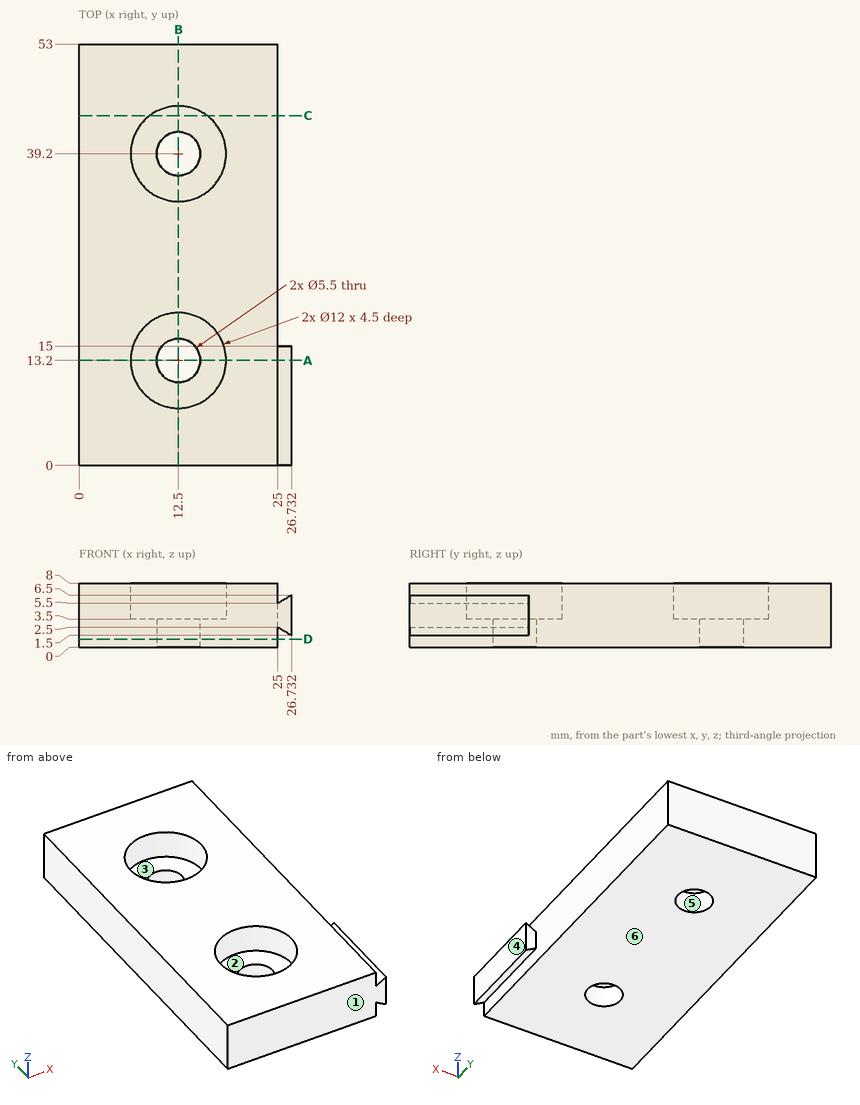
Could you check a few things on this drawing? It's one solid part, dimensions in mm from its lowest x, y, z. A direction names the side the tool comes from. Give positions to 0.01 mm unless a question says otherwise; leave off trailing zeros. Order: outer loops, then holes, each group sorted by start corner. A loop starts at its lowest first (then second) coordinate and runs counter-clockwise, first axis right, second up.
1. Suppose I cut it at C-C (y = 44). Write out the boundary of the cut face in (x, z).
Answers below:
outline: (0, 0) - (25, 0) - (25, 8) - (16.1, 8) - (16.1, 3.5) - (8.9, 3.5) - (8.9, 8) - (0, 8) - close
2. Thinking about a two-plate mould opening in X: for the marked faces 3, 4, 5 and 6, which applies, +X half, -X half, draft (parallel to the pull), parting line (faces both ways), or undercut?
Answers below:
face 3: undercut
face 4: +X half
face 5: undercut
face 6: draft
3. Suppose I cut it at A-A (y = 13.2). Write out the boundary of the cut face in (x, z).
Answers below:
outline: (0, 0) - (9.75, 0) - (9.75, 3.5) - (6.5, 3.5) - (6.5, 8) - (0, 8) - close; (15.25, 0) - (25, 0) - (25, 2.5) - (26.73, 1.5) - (26.73, 6.5) - (25, 5.5) - (25, 8) - (18.5, 8) - (18.5, 3.5) - (15.25, 3.5) - close
4. Suppose I cut it at B-B (x = 12.5). Write out the boundary of the cut face in (y, z).
Answers below:
outline: (0, 0) - (10.45, 0) - (10.45, 3.5) - (7.2, 3.5) - (7.2, 8) - (0, 8) - close; (15.95, 0) - (36.45, 0) - (36.45, 3.5) - (33.2, 3.5) - (33.2, 8) - (19.2, 8) - (19.2, 3.5) - (15.95, 3.5) - close; (41.95, 0) - (53, 0) - (53, 8) - (45.2, 8) - (45.2, 3.5) - (41.95, 3.5) - close
5. Suppose I cut it at D-D (z = 1). Write out the boundary of the cut face in (x, y), plus the area to 3 significant figures.
Answers below:
outline: (0, 0) - (25, 0) - (25, 53) - (0, 53) - close; hole circle Ø5.5 at (12.5, 13.2); hole circle Ø5.5 at (12.5, 39.2)
area: 1,280 mm2
6. Which directions (+Z, -Z, +X, -X, +Y, -Y) give clear straight access to the entire face, cutting with the end or side of a thin tool? Please do the marked faces 1 and 2.
Answers below:
face 1: +Z, -Z, +X, -X, -Y
face 2: +Z
7. For pin 1 (11 mm diameter, centred on x = 12.5, y = 39.2, fed in from +Z); pin 2 (3.5 mm diameter, centred on x = 12.5, y = 13.2, fed in from +Z); pin 3 (0.5 mm diameter, centred on x = 26, z = 3.5, fed in from +Y); pin 4 (1.5 mm diameter, centred on y = 28, z = 1.5, fed in from +X), each with a flat end and sliding along its axis, tell me the tip position at first contact or that it passes through.
Answers below:
pin 1: stops at z = 3.5
pin 2: passes through
pin 3: stops at y = 15
pin 4: stops at x = 25
8. I need wall thicknesses on L1, parallel to Y at x = 12.5, z = 7; L2, parallel to Y at x = 12.5, z = 2.15; L3, parallel to Z at x = 17, y = 16.5. Which ranges of each line are inside material? Lowest first, please.
Answers below:
L1: y = 0 to 7.2, 19.2 to 33.2, 45.2 to 53
L2: y = 0 to 10.45, 15.95 to 36.45, 41.95 to 53
L3: z = 0 to 3.5
